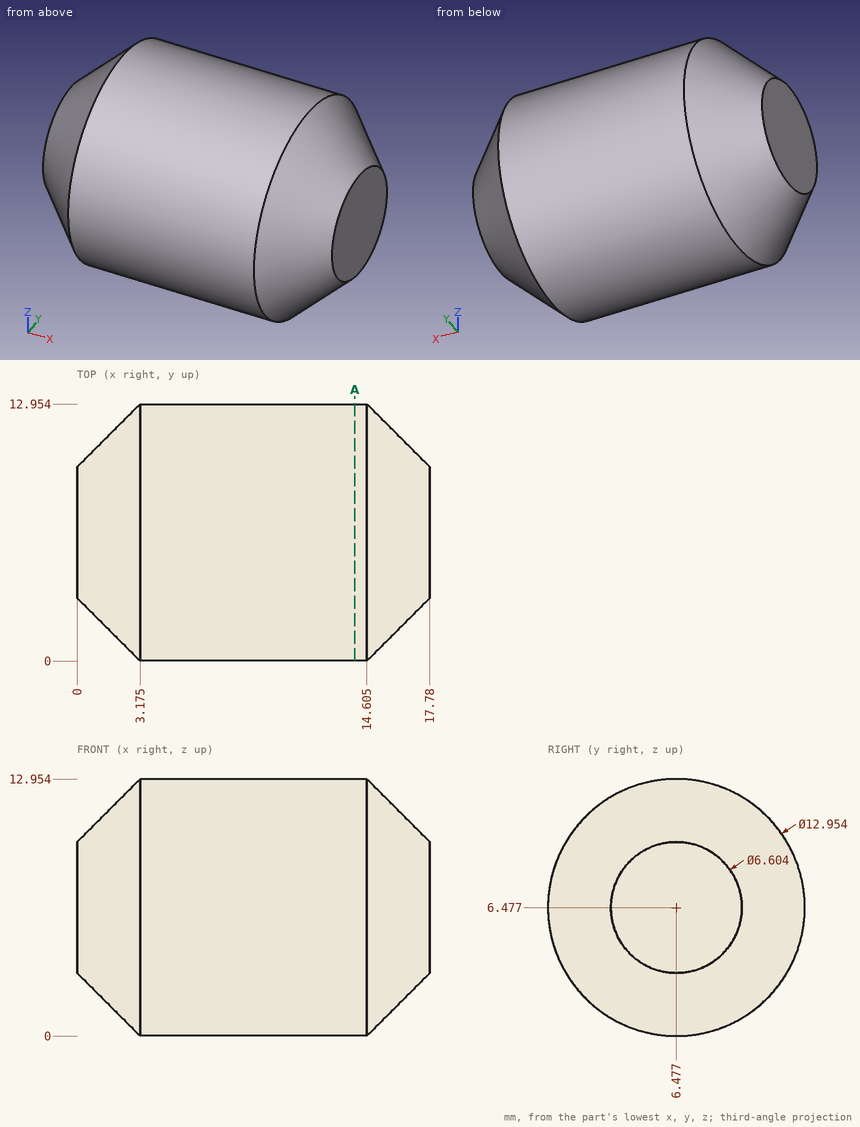
Print and shaded views of the part. All mm, measured from the part's lowest x, y and z. Coordinates: 2 decimals unless noted, no trailing zeros. Order: outer loops, then holes, each group sorted by start corner. A loop starts at its lowest first (then second) coordinate and runs counter-clockwise, first axis right, second up. Notation, with made-up numbers: (-7.75, -27.75) -> (13.25, -27.75) arc R25 cw to (13.25, -14.75) -> close; hole circle Ø11 at (-18, 41). An arc over 180 degrees is marked (long way). Answer as a JSON object with one key per item and string values. Group by question number.
1) Drill centre lines: L1, parallel to Y at x = 14, z = 10.5; L2, parallel to X at y = 11.5, z = 3.5; L3, parallel to Z at x = 13.5, y = 3.5. Where is each one in solid material? Low to high.
2) Cut at A-A, the plane x = 14. Write the cut outline in (y, z).
3) Flat gauge pins, fed straight in: pin 1 (5 mm diameter, centred on y = 2.5, z = 9, fed in from -X); pin 2 (4 mm diameter, centred on x = 11.5, z = 2, fed in from -Y). Where does each tip first touch, or does it go through?
Check values:
{
 "1": {"L1": "y = 1.4 to 11.55", "L2": "x = 2.54 to 15.24", "L3": "z = 0.72 to 12.23"},
 "2": {"outline": "circle Ø12.95 at (6.48, 6.48)"},
 "3": {"pin 1": "stops at x = 0", "pin 2": "stops at y = 0.49"}
}
